from build123d import *

# Parameters (mm, degrees)
EXTRUDE_1_DEPTH          = 55
EXTRUDE_1_DEPTH_BACK     = 55
EXTRUDE_2_DEPTH          = 140
EXTRUDE_2_DEPTH_BACK     = 140
SKETCH_2_W               = 4.5
SKETCH_2_H               = 90
FILLET_1_R               = 5
CUT_EXTRUDE_1_DEPTH      = 263.581415946
CUT_EXTRUDE_1_DEPTH_BACK = 263.581415946
SKETCH_3_R               = 7
SKETCH_3_R_2             = 1.65
SKETCH_3_R_3             = 2.5


with BuildPart() as part:
    # ｽｹｯﾁ1 → ﾎﾞｽ - 押し出し1 (new, two sides: drawn at the far end of the back side and taken through both)
    with BuildSketch(Plane.XY.offset(-EXTRUDE_1_DEPTH_BACK)):
        with BuildLine():
            Line((0, 0), (4.5, 0))
            Line((4.5, 0), (4.5, 45))
            Line((4.5, 45), (138.5, 45))
            ThreePointArc((138.5, 45), (141.681980515, 46.318019485), (143, 49.5))
            Line((143, 49.5), (143, 170))
            Line((143, 170), (138.5, 170))
            Line((138.5, 170), (138.5, 49.5))
            Line((138.5, 49.5), (4.5, 49.5))
            ThreePointArc((4.5, 49.5), (1.318019485, 48.181980515), (0, 45))
            Line((0, 45), (0, 0))
        make_face()
    extrude(amount=EXTRUDE_1_DEPTH + EXTRUDE_1_DEPTH_BACK)

    # ｽｹｯﾁ2 → ﾎﾞｽ - 押し出し2 (add, two sides: drawn at the far end of the back side and taken through both)
    with BuildSketch(Plane.XY.offset(-EXTRUDE_2_DEPTH_BACK)):
        with Locations((140.75, 125)):
            Rectangle(SKETCH_2_W, SKETCH_2_H)
    extrude(amount=EXTRUDE_2_DEPTH + EXTRUDE_2_DEPTH_BACK)

    # ﾌｨﾚｯﾄ1
    fillet_1_edges = [part.edges().sort_by_distance(p)[0] for p in [
        (2.25, 0, -55),
        (140.75, 80, -140),
        (140.75, 170, -140),
        (140.75, 80, 140),
        (140.75, 170, 140),
        (2.25, 0, 55),
    ]]
    fillet(fillet_1_edges, radius=FILLET_1_R)

    # ｽｹｯﾁ3 → ｶｯﾄ - 押し出し1 (cut, two sides: drawn at the far end of the back side and taken through both)
    with BuildSketch(Plane(origin=(0, 0, 0), x_dir=(0, 0, -1), z_dir=(1, 0, 0)).offset(-CUT_EXTRUDE_1_DEPTH_BACK)):
        with Locations((40, 20)):
            Circle(SKETCH_3_R)
        with Locations((-40, 20)):
            Circle(SKETCH_3_R)
        with Locations((0, 155)):
            Circle(SKETCH_3_R_2)
        with Locations((60, 155)):
            Circle(SKETCH_3_R_2)
        with Locations((-60, 155)):
            Circle(SKETCH_3_R_2)
        with Locations((120, 155)):
            Circle(SKETCH_3_R_2)
        with Locations((-120, 155)):
            Circle(SKETCH_3_R_2)
        with Locations((67.5, 129)):
            Circle(SKETCH_3_R_3)
        with Locations((-67.5, 129)):
            Circle(SKETCH_3_R_3)
        with Locations((97.5, 129)):
            Circle(SKETCH_3_R_3)
        with Locations((-97.5, 129)):
            Circle(SKETCH_3_R_3)
    extrude(amount=CUT_EXTRUDE_1_DEPTH + CUT_EXTRUDE_1_DEPTH_BACK, mode=Mode.SUBTRACT)


solid = part.part
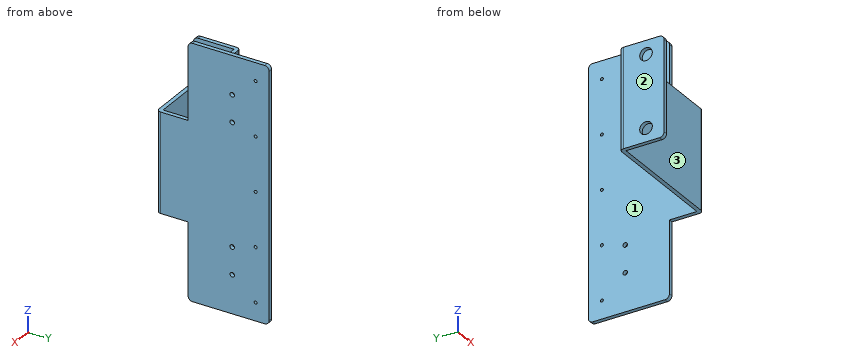
Check sheet for the modelled part. Datum: model origin and axes. Units: mm. Face numbers are marked on the shaded views. A direction names the side the tool comes from. Round coordinates to 2 decimals unless told otherwise and drop trailing zeros. Loops run counter-clockwise (first coordinate to the right, second up) from the corner with the lowest first, then second, coordinate; pieces in that order, holes last. Notation, with made-up numbers: M -27,42 L -2,42 A25 cw -2,62 Z; hole C 16.25,-22.75 d9. An arc over 180 degrees is marked long. One line per item, written item: value.
(1) Sectioned sample at C-C, the plane z = -21. Record the cut outline in (x, y).
Computed values:
outline: M 0,0 L 4.5,0 L 4.5,45 L 138.5,45 A4.5 ccw 143,49.5 L 143,170 L 138.5,170 L 138.5,49.5 L 4.5,49.5 A4.5 ccw 0,45 Z
(2) Depth check by flat-ended pin: pin 1 Ø4.5 at (y, z) = (155, -60) entering from -X; pin 2 Ø10 at (x, z) = (79.5, -57) entering from -Y; pin 3 Ø1.3 at (x, z) = (140.5, 92) entering from -Y. Enter the tip coordinate at first touch or a pass-through.
Computed values:
pin 1: stops at x = 138.5
pin 2: stops at y = 45
pin 3: stops at y = 80
(3) Sectioned sample at A-A, the plane y = 20. Record the cut outline in (x, z).
Computed values:
outline: M 0,-55 L 4.5,-55 L 4.5,-47 L 0,-47 Z; M 0,-33 L 4.5,-33 L 4.5,33 L 0,33 Z; M 0,47 L 4.5,47 L 4.5,55 L 0,55 Z
(4) Sectioned sample at B-B, the plane z = 40. Record the cut outline in (x, y).
Computed values:
outline: M 0,0 L 4.5,0 L 4.5,13 L 0,13 Z; M 0,27 L 4.5,27 L 4.5,45 L 138.5,45 A4.5 ccw 143,49.5 L 143,170 L 138.5,170 L 138.5,49.5 L 4.5,49.5 A4.5 ccw 0,45 Z
(5) Access from +Z, -Z, +X, -X, +Y, -Y to the whole of each face (thin tool, end or side, straight path). Record for the marked faces 1, 2 and 3.
Computed values:
face 1: +Z, -Z, -X, +Y
face 2: +Z, -Z, -X, +Y, -Y
face 3: +Z, -Z, +X, -Y
(6) Thickness scan on line 1 (Z direction, x = 140.7, y = 155); line 2 (Z direction, x = 2, y = 20); line 3 (Y direction, x = 140.3, z = 67.5). Record the ranges inside material, lowest first.
Computed values:
line 1: z = -140 to -121.65, -118.35 to -61.65, -58.35 to -1.65, 1.65 to 58.35, 61.65 to 118.35, 121.65 to 140
line 2: z = -55 to -47, -33 to 33, 47 to 55
line 3: y = 80 to 126.5, 131.5 to 170
(7) Sectioned sample at D-D, the plane y = 135. Record the cut outline in (x, z), then the cut area to 3 significant figures.
Computed values:
outline: M 138.5,-140 L 143,-140 L 143,140 L 138.5,140 Z
area: 1,260 mm^2
